Build history of the part. All positions in model axes, mm. A direction names the side the tool comes from. Coordinates: 2 decimals unless noted, no trailing zeros. Loops run counter-clockwise (first coordinate to the right, second up) from the corner with the lowest first, then second, coordinate; pieces in that order, holes last. Notation, with made-up numbers: (-11, -3) - (7, -3) arc R22 cw to (7, 13) - close; hole circle Ø7 at (31, 15). An arc over 180 degrees is marked (long way). One line per item, written item: value.
```python
from build123d import *

# Parameters (mm, degrees)
F3_DEPTH = 12
F4_SIZE  = 1
F5_SIZE  = 1.2


with BuildPart() as f1:
    # F0 (on Front) → F1 (revolve)
    with BuildSketch(Plane.XZ):
        Polygon((-6.7, 0), (-2.7, 0), (-2.7, 12), (-4.1, 12), (-4.1, 24), (-8.1, 24), (-8.1, 10), (-6.7, 6.153532), align=None)
    revolve(axis=Axis((0, 0, 10.296541), (0, 0, -1)))

    # F2 (on Top) → F3 (join)
    with BuildSketch(Plane.XY):
        with BuildLine():
            Line((-2, -1.813836), (-2, 1.813836))
            ThreePointArc((-2, 1.813836), (-2.7, 0), (-2, -1.813836))
        make_face()
    extrude(amount=F3_DEPTH)

    # F4
    f4_edges = [f1.edges().sort_by_distance(p)[0] for p in [
        (8.1, 0, 24),
        (6.7, 0, 0),
        (2.7, 0, 0),
        (-2, 0, 0),
        (4.1, 0, 24),
    ]]
    chamfer(f4_edges, length=F4_SIZE)

    # F5
    f5_edges = [f1.edges().sort_by_distance(p)[0] for p in [
        (8.1, 0, 10),
        (6.7, 0, 6.153532),
    ]]
    chamfer(f5_edges, length=F5_SIZE)


solid = f1.part
```
Item 1: Drop flat-ended pins along their axis: P1, Ø2, axis at y = 4.5, z = 14.5, coming from the -X side; P2, Ø2, axis at y = -3, z = 8.5, coming from the +X side; P3, Ø4.5, axis at x = 0, y = 0, coming from the -Z side; P4, Ø1, axis at x = 2, y = -3, coming from the -Z side. Give the stop position or say it passes through.
Check result:
P1: stops at x = -7.3
P2: stops at x = 7.41
P3: stops at z = 0.75
P4: stops at z = 0
Item 2: Cut at B-B, the plane z = 12.5. Write the cut outline in (x, y).
Check result:
outline: circle Ø16.2 at (0, 0); hole circle Ø8.2 at (0, 0)
Item 3: Tool access for faces 1 (the face through (-2, 0, 6)), 2 (the face through (0.534, 4.065, 17.577)), 3 (the face through (-2.5, 0, 0.5)): list every direction of +Z, -Z, +X, -X, +Y, -Y with a clear straight run to the whole face (end or side of a thin tool).
Check result:
face 1: +Z, -Z
face 2: +Z
face 3: -Z
Item 4: Probe probe 1 along X at (y, z) = (0, 4); probe 2 along Y at (x, z) = (0, 4.5); probe 3 along Y at (x, z) = (0, 18). List the from-to ranges inside material, lowest first. Write a range as from..to.
Check result:
probe 1: x = -6.7..-2, 2.7..6.7
probe 2: y = -6.7..-2.7, 2.7..6.7
probe 3: y = -8.1..-4.1, 4.1..8.1
Item 5: Cut at A-A, the plane z = 1.5. Write the cut outline in (x, y), then the cut area to 3 significant figures.
Check result:
outline: circle Ø13.4 at (0, 0); hole (-2, -1.81) arc R2.7 ccw (long way) to (-2, 1.81) - close
area: 120 mm^2
Item 6: Cut at C-C, the plane z = 7.75. Write the cut outline in (x, y).
Check result:
outline: circle Ø14.56 at (0, 0); hole (-2, -1.81) arc R2.7 ccw (long way) to (-2, 1.81) - close
Item 7: Pull direction Y, two halves, no side cores. Call faces 4 (the face through (-7.726, 2.433, 17.017)), 5 (the face through (2.9, 0.1, 0.8)), 6 (the face through (0, -4, 0)), 7 (the face through (1, -3, 12)): released by +Y, released by -Y, zero draft, split by the parting line, or undercut.
Check result:
face 4: split by the parting line
face 5: undercut
face 6: zero draft
face 7: undercut
